from build123d import *

# Parameters (mm, degrees)
F1_DEPTH = 5.08
F2_R     = 5.08
F3_R     = 5.08
F4_R     = 5.08
F5_R     = 5.08


with BuildPart() as f1:
    # F0 (on Front) → F1 (new body)
    with BuildSketch(Plane.XZ):
        Polygon((-101.6, 95.951064), (-101.6, -81.848936), (-50.8, -81.848936), (-50.8, -76.768936), (-96.52, -76.768936), (-96.52, 90.871064), (45.72, 90.871064), (45.72, -76.768936), (0, -76.768936), (0, -81.848936), (50.8, -81.848936), (50.8, 95.951064), align=None)
    extrude(amount=F1_DEPTH)

    # F2
    f2_edges = [f1.edges().sort_by_distance(p)[0] for p in [
        (-101.6, -2.54, 95.951064),
    ]]
    fillet(f2_edges, radius=F2_R)

    # F3
    f3_edges = [f1.edges().sort_by_distance(p)[0] for p in [
        (50.8, -2.54, 95.951064),
    ]]
    fillet(f3_edges, radius=F3_R)

    # F4
    f4_edges = [f1.edges().sort_by_distance(p)[0] for p in [
        (-101.6, -2.54, -81.848936),
    ]]
    fillet(f4_edges, radius=F4_R)

    # F5
    f5_edges = [f1.edges().sort_by_distance(p)[0] for p in [
        (50.8, -2.54, -81.848936),
    ]]
    fillet(f5_edges, radius=F5_R)


solid = f1.part
Model file for the job. Use its own axes, mm. A direction names the side the tool comes from. Round coordinates to 2 decimals unless told otherwise and drop trailing zeros. Order: outer loops, then holes, each group sorted by start corner. A loop starts at its lowest first (then second) coordinate and runs counter-clockwise, first axis right, second up. Notation, with made-up numbers: M -23.75,-6 L 23.25,-6 A17 ccw 23.25,1 Z; hole C -11,-6 d11. An arc over 180 degrees is marked long. Write each question's results on one line, items separated by ' | '. Start each with the question number.
(1) Saw through at A-A, the plane x = 11.5. Give the cut face in (y, z), then the cut area to 3 significant figures.
(2) Two-plate mould, pull along Z, no slides. Class faces 1 (the face through (23, -3, -81.849)), 2 (the face through (-101.6, -3, 8)), 3 (the face through (45.72, -3, 8)): pulls with the +Z half, pulls with the -Z half, needs draft (parallel to the pull), parting line crosses it, or undercut.
(3) Drop flat-ended pins along their axis: pin 1 (1.5 mm diameter, centred on y = -3, z = -78, fed in from -X); pin 2 (2.5 mm diameter, centred on y = -3, z = -79.5, fed in from +X); pin 3 (1.5 mm diameter, centred on x = -33.5, y = -4, fed in from -Z). Give the stop position or say it passes through.
(4) Saw through at C-C, the plane y = -4.2. Give the cut face in (x, z).
(5) Saw through at D-D, the plane x = -5.5. Give the cut face in (y, z).
(6) Which spindle directions (+Z, -Z, +X, -X, +Y, -Y) get a long thin tool onto all of the face, cutting with end or side? Do faces 4 (the face through (-26, -3, 90.871)), 5 (the face through (-50.8, -3, -79)), 6 (the face through (-24, -3, 95.951)). Say none if no direction does.
(7) Saw through at B-B, the plane z = -18. Give the cut face in (x, y), then the cut area to 3 significant figures.
(8) Probe probe 1 along X at (y, z) = (-3.15, -37.5); probe 2 along Z at (x, y) = (26, -1.65); probe 3 along Z at (x, y) = (-37, -1.15). List the from-to ranges inside material, lowest first. Write a range as from..to.
Established:
1) outline: M -5.08,-81.85 L 0,-81.85 L 0,-76.77 L -5.08,-76.77 Z; M -5.08,90.87 L 0,90.87 L 0,95.95 L -5.08,95.95 Z | area: 51.6 mm^2
2) face 1: pulls with the -Z half | face 2: needs draft | face 3: undercut
3) pin 1: stops at x = -101.58 | pin 2: stops at x = 50.58 | pin 3: stops at z = 90.87
4) outline: M -101.6,-76.77 A5.08 ccw -96.52,-81.85 L -50.8,-81.85 L -50.8,-76.77 L -96.52,-76.77 L -96.52,90.87 L 45.72,90.87 L 45.72,-76.77 L 0,-76.77 L 0,-81.85 L 45.72,-81.85 A5.08 ccw 50.8,-76.77 L 50.8,90.87 A5.08 ccw 45.72,95.95 L -96.52,95.95 A5.08 ccw -101.6,90.87 Z
5) outline: M -5.08,90.87 L 0,90.87 L 0,95.95 L -5.08,95.95 Z
6) face 4: +Y, -Y | face 5: -Z, +Y, -Y | face 6: +Z, +X, -X, +Y, -Y
7) outline: M -101.6,-5.08 L -96.52,-5.08 L -96.52,0 L -101.6,0 Z; M 45.72,-5.08 L 50.8,-5.08 L 50.8,0 L 45.72,0 Z | area: 51.6 mm^2
8) probe 1: x = -101.6..-96.52, 45.72..50.8 | probe 2: z = -81.85..-76.77, 90.87..95.95 | probe 3: z = 90.87..95.95
